```python
from build123d import *

# Parameters (mm, degrees)
SKETCH1_R                = 11
SKETCH1_R_2              = 5
SKETCH1_R_3              = 1.5
BOSS_EXTRUDE1_DEPTH      = 3
SKETCH2_R                = 5
SKETCH2_R_2              = 4
BOSS_EXTRUDE2_DEPTH      = 8
BOSS_EXTRUDE2_DEPTH_BACK = 2


with BuildPart() as part:
    # Sketch1 → Boss-Extrude1 (new body)
    with BuildSketch(Plane(origin=(0, 0, 0), x_dir=(1, 0, 0), z_dir=(0, 1, 0))):
        Circle(SKETCH1_R)
        Circle(SKETCH1_R_2, mode=Mode.SUBTRACT)
        with Locations((-5.75, 5.75)):
            Circle(SKETCH1_R_3, mode=Mode.SUBTRACT)
        with Locations((5.75, 5.75)):
            Circle(SKETCH1_R_3, mode=Mode.SUBTRACT)
        with Locations((5.75, -5.75)):
            Circle(SKETCH1_R_3, mode=Mode.SUBTRACT)
        with Locations((-5.75, -5.75)):
            Circle(SKETCH1_R_3, mode=Mode.SUBTRACT)
    extrude(amount=BOSS_EXTRUDE1_DEPTH)

    # Sketch2 → Boss-Extrude2 (add, two sides)
    with BuildSketch(Plane(origin=(0, 0, 0), x_dir=(1, 0, 0), z_dir=(0, 1, 0))) as boss_extrude2_sk:
        Circle(SKETCH2_R)
        Circle(SKETCH2_R_2, mode=Mode.SUBTRACT)
    extrude(amount=BOSS_EXTRUDE2_DEPTH)
    extrude(boss_extrude2_sk.sketch, amount=-BOSS_EXTRUDE2_DEPTH_BACK)


solid = part.part
```
For this review, take the finished solid that the model builds, in its own axes (mm). A direction names the side the tool comes from. Round coordinates to 2 decimals unless told otherwise and drop trailing zeros. Write each loop counter-clockwise with the first axis right and the second up, starting at its lowest first coordinate (ties: lowest second). Pieces come first, ordered by that corner, then holes. Notation, with made-up numbers: (39.25, -7.5) -> (50.25, -7.5) arc R6 cw to (50.25, 0.5) -> close; hole circle Ø3 at (-29, -36). An arc over 180 degrees is marked (long way). Use one line per item in the form item = value.
Q1. Clearance check with flat-ended pins moving along their axes: pin 1 Ø8 at (x, z) = (-3, -0.5) entering from -Y; pin 2 Ø2 at (y, z) = (0, -3.5) entering from +X; pin 3 Ø2 at (x, y) = (7.5, 1.5) entering from -Z; pin 4 Ø4 at (x, z) = (-5.75, -5.75) entering from +Y. State where each tip first meets the part, or that it passes through.
Resolved:
pin_1 = -2
pin_2 = 10.71
pin_3 = -8.87
pin_4 = 3
Q2. Consider section A-A (x = 0). State the section outline as (y, z) points, then the cut area to 3 significant figures.
Resolved:
outline = (-2, -5) -> (0, -5) -> (0, -11) -> (3, -11) -> (3, -5) -> (8, -5) -> (8, -4) -> (-2, -4) -> close; (-2, 4) -> (8, 4) -> (8, 5) -> (3, 5) -> (3, 11) -> (0, 11) -> (0, 5) -> (-2, 5) -> close
area = 56.0 mm²
Q3. Consider section C-C (x = 5.75). State the section outline as (y, z) points, then the cut area to 3 significant figures.
Resolved:
outline = (0, -9.38) -> (3, -9.38) -> (3, -7.25) -> (0, -7.25) -> close; (0, -4.25) -> (3, -4.25) -> (3, 4.25) -> (0, 4.25) -> close; (0, 7.25) -> (3, 7.25) -> (3, 9.38) -> (0, 9.38) -> close
area = 38.3 mm²
Q4. Machinability: for faces 4 (the cylindrical face through (-1.08, -0.99, 4.88)), 5 (the cylindrical face through (-6.94, 1.48, -4.84)), 6 (the cylindrical face through (-1.08, 5.46, 4.88)), which of the approach directions +Z, -Z, +X, -X, +Y, -Y give a long, thin tool a straight path to every point of the face, cutting with its end or side? Answer none if there is none.
Resolved:
face_4 = -Y
face_5 = +Y, -Y
face_6 = +Y
Q5. The part is to be moulded in two halves that separate along Z. For faces 1 (the flat face through (2, 3, 5)), 2 (the cylindrical face through (-2.38, 1.48, 10.74)), 3 (the cylindrical face through (-6.94, 1.48, 6.66)), say which applies: released by +Z, released by -Z, zero draft, split by the parting line, or undercut.
Resolved:
face_1 = zero draft
face_2 = split by the parting line
face_3 = undercut
Q6. Consider section B-B (z = -1.5). State the section outline as (x, y) points, then the cut area to 3 significant figures.
Resolved:
outline = (-10.9, 0) -> (-4.77, 0) -> (-4.77, -2) -> (-3.71, -2) -> (-3.71, 8) -> (-4.77, 8) -> (-4.77, 3) -> (-10.9, 3) -> close; (3.71, -2) -> (4.77, -2) -> (4.77, 0) -> (10.9, 0) -> (10.9, 3) -> (4.77, 3) -> (4.77, 8) -> (3.71, 8) -> close
area = 58.0 mm²
Q7. To check wall thickness, follow probe 1 along Z at (x, y) = (0, 0.75); probe 2 along Z at (x, y) = (-5.75, 1.6); probe 3 along Z at (x, y) = (0, 6.25). State the ranges of each line that lie inside material, in increasing order. Write a range as from..to.
Resolved:
probe_1 = -11..-4, 4..11
probe_2 = -9.38..-7.25, -4.25..4.25, 7.25..9.38
probe_3 = -5..-4, 4..5
Q8. Consider section D-D (y = 1.5). State the section outline as (x, z) points, then the cut area to 3 significant figures.
Resolved:
outline = circle Ø22 at (0, 0); hole circle Ø3 at (-5.75, -5.75); hole circle Ø3 at (-5.75, 5.75); hole circle Ø8 at (0, 0); hole circle Ø3 at (5.75, -5.75); hole circle Ø3 at (5.75, 5.75)
area = 302 mm²
